from build123d import *

# Parameters (mm, degrees)
BOSS_EXTRUDE1_DEPTH = 3
CHAMFER1_SIZE       = 2
FILLET1_R           = 1


with BuildPart() as part:
    # Sketch1 → Boss-Extrude1 (new body)
    with BuildSketch(Plane.XY):
        Polygon((0, 0), (25, 0), (25, 5), (22.5, 5), (22.5, 8), (17.5, 8), (17.5, 5), (7.5, 5), (7.5, 8), (2.5, 8), (2.5, 5), (0, 5), align=None)
    extrude(amount=BOSS_EXTRUDE1_DEPTH)

    # Chamfer1
    chamfer1_edges = [part.edges().sort_by_distance(p)[0] for p in [
        (25, 0, 1.5),
        (0, 0, 1.5),
    ]]
    chamfer(chamfer1_edges, length=CHAMFER1_SIZE)

    # Fillet1
    fillet1_edges = [part.edges().sort_by_distance(p)[0] for p in [
        (25, 2, 1.5),
        (2, 0, 1.5),
        (23, 0, 1.5),
        (0, 2, 1.5),
    ]]
    fillet(fillet1_edges, radius=FILLET1_R)


solid = part.part
The listing builds one solid part. Answer for the finished solid, in the listing's coordinates (mm). A direction names the side the tool comes from. Round coordinates to 2 decimals unless told otherwise and drop trailing zeros. Write each loop counter-clockwise with the first axis right and the second up, starting at its lowest first coordinate (ties: lowest second). Pieces come first, ordered by that corner, then holes. Notation, with made-up numbers: M -35,56.5 L 18,56.5 A24 cw 18,94.5 Z; hole C 3,46 d2. An arc over 180 degrees is marked long. Write each question's results on one line, items separated by ' | '. Start each with the question number.
Item 1: Straight lines are drawn through the part: L1, parallel to X at y = 5.5, z = 2.35; L2, parallel to Y at x = 15, z = 0.95; L3, parallel to X at y = 1.75, z = 1.95. For each, find the intervals that lie inside material, in ascending order. Write a range as [from, to].
Item 2: A cutting plane is placed at B-B on z = 0.35. Write down the section's boundary in (x, y).
Item 3: For a pull along X with two mould halves and no side action, classify faces 6 (the face through (5, 8, 1)), 7 (the face through (2.5, 7, 1)), 8 (the face through (7.5, 6, 1)), 9 (the face through (13, 5, 1)) as pulls with the +X half, pulls with the -X half, needs draft (parallel to the pull), parting line crosses it, or undercut.
Item 4: For faces 1 (the face through (22.5, 6, 1)), 2 (the face through (1, 5, 1)), 3 (the face through (12, 0, 1)), 4 (the face through (17.5, 7, 1)), 5 (the face through (12, 3, 0)), determine the directions among +Z, -Z, +X, -X, +Y, -Y from which every point of the face is accessible in a straight line to the end or side of a thin tool.
Item 5: A cutting plane is placed at D-D on x = 14.25. Write down the section's boundary in (y, z), and give its area (3 significant figures).
Item 6: Flat-ended cylindrical pins translate along their axes: pin 1 Ø1 at (y, z) = (2, 0.5) entering from -X; pin 2 Ø1.2 at (x, z) = (1.5, 1) entering from +Y; pin 3 Ø1.5 at (y, z) = (6.5, 1.5) entering from -X. Find the tip coordinate at first contact, or state that the pin passes through.
Item 7: A cutting plane is placed at A-A on y = 5.75. Write down the section's boundary in (x, z).
Item 8: A cutting plane is placed at C-C on x = 23.75. Write down the section's boundary in (y, z).
Check sheet entries:
1) L1: [2.5, 7.5], [17.5, 22.5] | L2: [0, 5] | L3: [0.25, 24.75]
2) outline: M 0,2.41 A1 ccw 0.29,1.71 L 1.71,0.29 A1 ccw 2.41,0 L 22.59,0 A1 ccw 23.29,0.29 L 24.71,1.71 A1 ccw 25,2.41 L 25,5 L 22.5,5 L 22.5,8 L 17.5,8 L 17.5,5 L 7.5,5 L 7.5,8 L 2.5,8 L 2.5,5 L 0,5 Z
3) face 6: needs draft | face 7: pulls with the -X half | face 8: undercut | face 9: undercut
4) face 1: +Z, -Z, +X, +Y | face 2: +Z, -Z, -X, +Y | face 3: +Z, -Z, +X, -X, -Y | face 4: +Z, -Z, +Y | face 5: -Z, +X, -X, +Y, -Y
5) outline: M 0,0 L 5,0 L 5,3 L 0,3 Z | area: 15.0 mm²
6) pin 1: x = 0 | pin 2: y = 5 | pin 3: x = 2.5
7) outline: M 2.5,0 L 7.5,0 L 7.5,3 L 2.5,3 Z; M 17.5,0 L 22.5,0 L 22.5,3 L 17.5,3 Z
8) outline: M 0.75,0 L 5,0 L 5,3 L 0.75,3 Z
